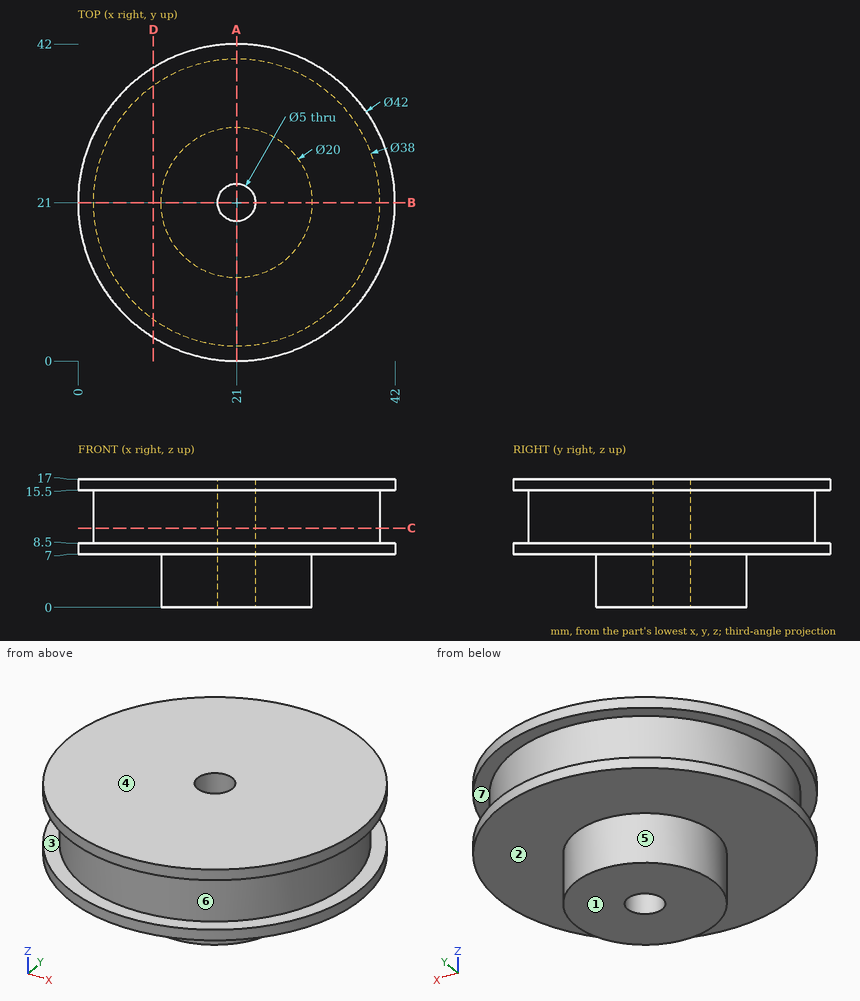
Study the drawing (mm; zero at the part's minimum x, y, z) and answer. A direction names the side the tool comes from. Give positions to 0.01 mm unless a question says otherwise; leave off trailing zeros. Order: outer loops, then holes, each group sorted by start corner. A loop starts at its lowest first (then second) coordinate and runs counter-clockwise, first axis right, second up.
1. Section D-D, the plane x = 10 is taken. Determine the outline of the cut face in (y, z).
Result sheet:
outline: (3.11, 7) - (38.89, 7) - (38.89, 8.5) - (36.49, 8.5) - (36.49, 15.5) - (38.89, 15.5) - (38.89, 17) - (3.11, 17) - (3.11, 15.5) - (5.51, 15.5) - (5.51, 8.5) - (3.11, 8.5) - close
2. Section C-C, the plane z = 10.5 is taken. Determine the outline of the cut face in (x, y).
Result sheet:
outline: circle Ø38 at (21, 21); hole circle Ø5 at (21, 21)
3. Each of these flat-tipped pins is pushed along its axis until it touches: P1, Ø5, axis at x = 5.5, z = 7, coming from the -Y side; P2, Ø6, axis at x = 21, y = 21, coming from the -Z side; P3, Ø1, axis at x = 25.5, y = 35, coming from the -Z side; P4, Ø2, axis at x = 9.5, z = 7, coming from the +Y side. Where does it stop, or does it pass through?
Result sheet:
P1: stops at y = 4.51
P2: stops at z = 0
P3: stops at z = 7
P4: stops at y = 39.19
4. For the marked faces 1, 2 and 3, determine the directions among +Z, -Z, +X, -X, +Y, -Y from which every point of the face is accessible in a straight line to the end or side of a thin tool.
Result sheet:
face 1: -Z, +X, -X, +Y, -Y
face 2: -Z
face 3: none
5. Straight lines are drawn through the part: L1, parallel to Y at x = 21, z = 11.75; L2, parallel to Z at x = 12, y = 38; L3, parallel to Y at x = 21, z = 5. For each, find the intervals that lie inside material, in ascending order.
Result sheet:
L1: y = 2 to 18.5, 23.5 to 40
L2: z = 7 to 8.5, 15.5 to 17
L3: y = 11 to 18.5, 23.5 to 31
6. Section A-A, the plane x = 21 is taken. Determine the outline of the cut face in (y, z).
Result sheet:
outline: (0, 7) - (11, 7) - (11, 0) - (18.5, 0) - (18.5, 17) - (0, 17) - (0, 15.5) - (2, 15.5) - (2, 8.5) - (0, 8.5) - close; (23.5, 0) - (31, 0) - (31, 7) - (42, 7) - (42, 8.5) - (40, 8.5) - (40, 15.5) - (42, 15.5) - (42, 17) - (23.5, 17) - close
7. The mould has two halves that part along Z. Classify the marked faces 4, 5, 6 and 7: released by +Z, released by -Z, zero draft, split by the parting line, or undercut.
Result sheet:
face 4: released by +Z
face 5: zero draft
face 6: undercut
face 7: undercut
